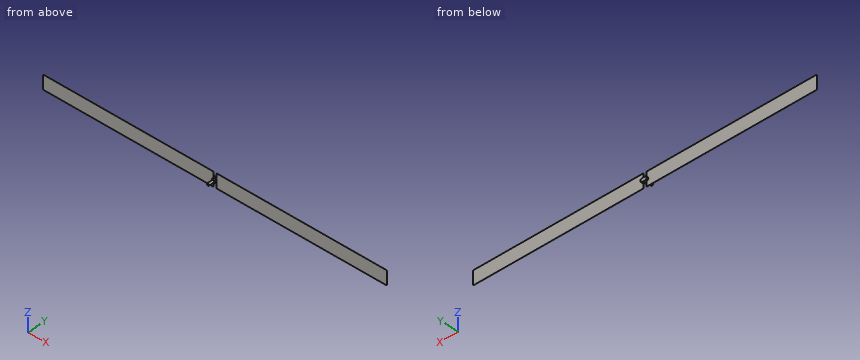
```python
from build123d import *

# Parameters (mm, degrees)
SKETCH1_R           = 0.37702405
SKETCH1_R_2         = 0.3
BOSS_EXTRUDE1_DEPTH = 2
SKETCH2_W           = 1
SKETCH2_H           = 1
BOSS_EXTRUDE2_DEPTH = 0.7
BOSS_EXTRUDE3_DEPTH = 0.5
SKETCH4_R           = 0.1
CUT_EXTRUDE2_DEPTH  = 0.4
BOSS_EXTRUDE4_DEPTH = 0.01


with BuildPart() as part:
    # Sketch1 → Boss-Extrude1 (new body)
    with BuildSketch(Plane(origin=(0, 0, 0), x_dir=(1, 0, 0), z_dir=(0, 1, 0))):
        Circle(SKETCH1_R)
        Circle(SKETCH1_R_2, mode=Mode.SUBTRACT)
    extrude(amount=BOSS_EXTRUDE1_DEPTH)

    # Sketch2 → Boss-Extrude2 (add)
    with BuildSketch(Plane(origin=(0, 2, 0), x_dir=(1, 0, 0), z_dir=(0, 1, 0))):
        Rectangle(SKETCH2_W, SKETCH2_H)
    extrude(amount=BOSS_EXTRUDE2_DEPTH)

    # Sketch3 → Boss-Extrude3 (add)
    with BuildSketch(Plane(origin=(0, 2.7, 0), x_dir=(1, 0, 0), z_dir=(0, 1, 0))):
        with BuildLine():
            Line((-0.5, 0.662390112), (0.5, 0.662390112))
            ThreePointArc((0.5, 0.662390112), (1.162390112, 0), (0.5, -0.662390112))
            Line((0.5, -0.662390112), (-0.5, -0.662390112))
            ThreePointArc((-0.5, -0.662390112), (-1.162390112, 0), (-0.5, 0.662390112))
        make_face()
    extrude(amount=BOSS_EXTRUDE3_DEPTH)

    # Sketch4 → Cut-Extrude2 (cut)
    with BuildSketch(Plane(origin=(0, 3.2, 0), x_dir=(1, 0, 0), z_dir=(0, 1, 0))):
        with Locations((-0.941559445, 0)):
            Circle(SKETCH4_R)
        with Locations((0.941559445, 0)):
            Circle(SKETCH4_R)
    extrude(amount=-CUT_EXTRUDE2_DEPTH, mode=Mode.SUBTRACT)

    # Sketch5 → Boss-Extrude4 (add)
    with BuildSketch(Plane.XZ.offset(-2.7)):
        with BuildLine():
            Line((0.8, -2.5), (60.8, -2.5))
            ThreePointArc((60.8, -2.5), (61.012132034, -2.412132034), (61.1, -2.2))
            Line((61.1, -2.2), (61.1, 2.2))
            ThreePointArc((61.1, 2.2), (61.012132034, 2.412132034), (60.8, 2.5))
            Line((60.8, 2.5), (0.5, 2.5))
            Line((0.5, 2.5), (0.5, -2.2))
            ThreePointArc((0.5, -2.2), (0.587867966, -2.412132034), (0.8, -2.5))
        make_face()
        with BuildLine():
            Line((-0.8, 2.5), (-60.8, 2.5))
            ThreePointArc((-60.8, 2.5), (-61.012132034, 2.412132034), (-61.1, 2.2))
            Line((-61.1, 2.2), (-61.1, -2.2))
            ThreePointArc((-61.1, -2.2), (-61.012132034, -2.412132034), (-60.8, -2.5))
            Line((-60.8, -2.5), (-0.8, -2.5))
            Line((-0.8, -2.5), (-0.5, -2.5))
            Line((-0.5, -2.5), (-0.5, -2.2))
            Line((-0.5, -2.2), (-0.5, 2.2))
            ThreePointArc((-0.5, 2.2), (-0.587867966, 2.412132034), (-0.8, 2.5))
        make_face()
    extrude(amount=BOSS_EXTRUDE4_DEPTH)


solid = part.part
```
Check sheet for the modelled part. Datum: model origin and axes. Units: mm. Coordinates: 2 decimals unless noted, no trailing zeros. Order: outer loops, then holes, each group sorted by start corner. A loop starts at its lowest first (then second) coordinate and runs counter-clockwise, first axis right, second up. Notation, with made-up numbers: (-8, -36) -> (37, -36) arc R6 cw to (37, -26) -> close; hole circle Ø6 at (18.25, 23). An arc over 180 degrees is marked (long way). Write item = value, one per line. Start each with the question number.
1) Material ranges on L1, parallel to X at y = 2.65, z = -0.2, recorded low to high.
2) Go/stop test with flat-tipped pins: P1, Ø2.5, axis at x = 22, z = 1, coming from the -Y side; P2, Ø2.5, axis at x = -20.5, z = 0, coming from the +Y side; P3, Ø0.6, axis at x = 0, y = 3, coming from the -Z side. Record where each tip stops, or that it passes through.
3) Cross-section at A-A (y = 0.5). Enter the section's corners in (x, z).
Ans:
q1.L1 = -0.5 to 0.5
q2.P1 = 2.69
q2.P2 = 2.7
q2.P3 = -0.66
q3.outline = circle Ø0.75 at (0, 0); hole circle Ø0.6 at (0, 0)
